Can you work these out from the model? Positions are in its coordinate system, mm. Face numbers are marked on the shaded views. A direction names the side the tool comes from. Coordinates: 2 decimals unless noted, no trailing zeros. Order: outer loops, then holes, each group sorted by start corner. A loop starts at its lowest first (then second) coordinate and runs counter-clockwise, first axis right, second up. Notation, with made-up numbers: (28, 15.25) - (67, 15.25) arc R18 ccw to (67, 35.25) - close; hole circle Ø10 at (-27, 69). An arc over 180 degrees is marked (long way). Return JSON: item names as keys, results as strings. Group by question number.
1) For pin 1 Ø5 at (x, y) = (16, 0.5) entering from -Z; pin 2 Ø1 at (x, z) = (-2.5, 1.5) entering from -Y, each with a flat end and sliding along its axis, tell me the tip position at first contact or that it passes through.
2) Imagine slicing it at A-A (x = 15.5). Write out the boundary of the cut face in (y, z), and give its area (3 significant figures).
3) Imagine slicing it at B-B (y = -1.5). Write out the boundary of the cut face in (x, z).
4) If I drill on line 1 along Y through (x, z) = (15.75, 0.85); line 2 along Y through (x, z) = (17.25, 0.8); line 3 along X through (y, z) = (-3, 1.6), over which ranges is the centre line in solid material (lowest first)?
5) Which directions (+Z, -Z, +X, -X, +Y, -Y) give clear straight access to the entire face, cutting with the end or side of a thin tool? Please do the marked faces 1 and 2.
6) Imagine slicing it at C-C (z = 0.35). Write out the boundary of the cut face in (x, y) (3 decimals).
7) If we mould it in two halves opening along X, with no side actions, what happens to the marked faces 3, 4 and 5? For each: pulls with the +X half, pulls with the -X half, needs draft (parallel to the pull), parting line crosses it, or undercut.
Autodesk Inventor part; units mm, degrees
ref_plane "YZ Plane" through (0, 0, 0) normal (1, 0, 0) x (0, 1, 0)
ref_plane "XZ Plane" through (0, 0, 0) normal (0, 1, 0) x (-1, 0, 0)
ref_plane "XY Plane" through (0, 0, 0) normal (0, 0, 1) x (1, 0, 0)
sketch "Sketch1" plane through (0, 0, 0) normal (0, 0, 1) x (1, 0, 0)
  line L0 (1.5, -5.75) -> (-1.9843, -5.75)
  line L1 (0, 0) -> (1.5, 0)
  line L2 (1.5, 0) -> (1.5, 5.75)
  line L3 (-16, 5.75) -> (1.5, 5.75)
  line L4 (-16, 3.21) -> (-16, 5.75)
  line L5 (0, 3.21) -> (-16, 3.21)
  line L6 (0, 2.75) -> (0, 3.21)
  line L7 (0, 2.75) -> (-1.9843, 2.75)
  arc A0 (-1.9843, 2.75) -> (-3.3072, 2.25) centre (-1.9843, 0.75) ccw
  arc A1 (-3.3072, 2.25) -> (-3.3072, -5.25) centre (0, -1.5) ccw
  arc A2 (-3.3072, -5.25) -> (-1.9843, -5.75) centre (-1.9843, -3.75) ccw
  line L8 (1.5, -5.75) -> (-1.9843, -5.75)
  line L9 (1.5, -5.75) -> (1.5, -3)
  line L10 (1.5, -3) -> (0, -3)
  line L11 (0, -3) -> (0, -2.5)
  line L12 (0, -2.5) -> (-1.5, -2.5)
  arc A3 (-1.5, -0.5) -> (-1.5, -2.5) centre (-1.5, -1.5) ccw
  line L13 (-1.5, -0.5) -> (0, -0.5)
  line L14 (0, -0.5) -> (0, 0)
  line L15 (15, -3) -> (13.5, -3)
  line L16 (13.5, -5.75) -> (13.5, -3)
  line L17 (13.5, -5.75) -> (16.9843, -5.75)
  arc A4 (16.9843, -5.75) -> (18.3072, -5.25) centre (16.9843, -3.75) ccw
  arc A5 (18.3072, -5.25) -> (18.3072, 2.25) centre (15, -1.5) ccw
  arc A6 (18.3072, 2.25) -> (16.9843, 2.75) centre (16.9843, 0.75) ccw
  line L18 (15, 2.75) -> (16.9843, 2.75)
  line L19 (15, 2.75) -> (15, 3.21)
  line L20 (31, 3.21) -> (15, 3.21)
  line L21 (31, 3.21) -> (31, 5.75)
  line L22 (13.5, 5.75) -> (31, 5.75)
  line L23 (13.5, 0) -> (13.5, 5.75)
  line L24 (13.5, 0) -> (15, 0)
  line L25 (15, 0) -> (15, -0.5)
  line L26 (15, -0.5) -> (16.5, -0.5)
  arc A7 (16.5, -2.5) -> (16.5, -0.5) centre (16.5, -1.5) ccw
  line L27 (16.5, -2.5) -> (15, -2.5)
  line L28 (15, -2.5) -> (15, -3)
  line L29 (14.7679, -0.5) -> (15, -0.366)
  line L30 (15, 0) -> (15, -0.366)
  line L31 (13.5, 0) -> (15, 0)
  line L32 (13.5, -3) -> (13.5, 0)
  line L33 (15, -3) -> (13.5, -3)
  line L34 (15, -2.634) -> (15, -3)
  line L35 (15, -2.634) -> (14.7679, -2.5)
  line L36 (14.7679, -2.5) -> (14.7679, -0.5)
  line L37 (0, -0.366) -> (0.2321, -0.5)
  line L38 (0.2321, -0.5) -> (0.2321, -2.5)
  line L39 (0.2321, -2.5) -> (0, -2.634)
  line L40 (0, -2.634) -> (0, -3)
  line L41 (0, -3) -> (1.5, -3)
  line L42 (1.5, 0) -> (1.5, -3)
  line L43 (1.5, 0) -> (0, 0)
  line L44 (0, 0) -> (0, -0.366)
  line L45 (20, -1.5) -> (20, -5.75)
  line L46 (13.5, -5.75) -> (20, -5.75)
  line L47 (13.5, -5.75) -> (-1.9843, -5.75)
  line L48 (-5, -1.5) -> (-5, -5.75)
  line L49 (-5, -5.75) -> (-1.9843, -5.75)
  line L50 (20, -5.75) -> (-5, -5.75)
  line L51 (-5, -5.75) -> (-5, 5.75)
  line L52 (-5, 5.75) -> (20, 5.75)
  line L53 (20, 5.75) -> (20, -5.75)
extrude "Extrusion1" add sketch "Sketch1" along normal blind 2 contours L0 A2 A1 A0 L7 L6 L5 L51 L3 L2 L1 L14 L13 A3 L12 L11 L10 L9 | L9 L42 L2 L52 L23 L32 L16 L47 | L49 L48 A1 A2 | L10 L11 L39 L38 L37 L14 L1 L42 | L16 L15 L28 L27 A7 L26 L25 L24 L23 L22 L53 L20 L19 L18 A6 A5 A4 L17 | L32 L24 L25 L29 L36 L35 L28 L15 | A4 A5 L45 L46 | L51 L5 L6 L7 A0 A1 | A5 A6 L18 L19 L20 L53
fillet "Fillet1" radius 3.175 2 edges at (-5, -5.75, 1) (20, -5.75, 1)
properties part number "N20Bracklet-Holder"
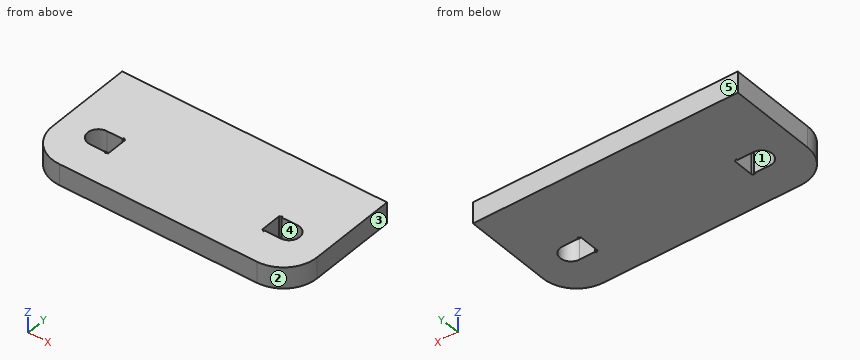
Calculated:
{
 "1": {"pin 1": "z = 0", "pin 2": "y = -5.75"},
 "2": {"outline": "(-5.75, 0) - (-2.5, 0) - (-2.5, 2) - (-5.75, 2) - close; (-0.5, 0) - (5.75, 0) - (5.75, 2) - (-0.5, 2) - close", "area": "19.0 mm2"},
 "3": {"outline": "(-5, 0) - (-2.5, 0) - (-2.5, 2) - (-5, 2) - close; (0.23, 0) - (14.77, 0) - (14.77, 2) - (0.23, 2) - close; (17.5, 0) - (20, 0) - (20, 2) - (17.5, 2) - close"},
 "4": {"line 1": "-5.75 to -2.5, -0.5 to 5.75", "line 2": "-5.72 to -2.16, -0.84 to 5.75", "line 3": "-4.97 to 19.97"},
 "5": {"face 1": "+Z, -Z", "face 2": "+Z, -Z, +X, -Y"},
 "6": {"outline": "(-5, -2.575) arc R3.175 ccw to (-1.825, -5.75) - (16.825, -5.75) arc R3.175 ccw to (20, -2.575) - (20, 5.75) - (-5, 5.75) - close; hole (-1.5, -2.5) - (0, -2.5) - (0, -2.634) - (0.232, -2.5) - (0.232, -0.5) - (0, -0.366) - (0, -0.5) - (-1.5, -0.5) arc R1 ccw to start; hole (14.768, -2.5) - (15, -2.634) - (15, -2.5) - (16.5, -2.5) arc R1 ccw to (16.5, -0.5) - (15, -0.5) - (15, -0.366) - (14.768, -0.5) - close"},
 "7": {"face 3": "pulls with the +X half", "face 4": "undercut", "face 5": "needs draft"}
}
